from build123d import *

# Parameters (mm, degrees)
F0_R     = 2
F0_R_2   = 39
F0_R_3   = 34
F1_DEPTH = 5
F2_R     = 38
F2_R_2   = 47
F3_DEPTH = 0.5


# Not quite as in the source:
# - a fillet or chamfer that OpenCascade refuses, or shapes differently, is made with other operations: its cross-section is extruded or revolved along the edge and cut away or added


with BuildPart() as f1:
    # F0 (on Front) → F1 (new body)
    with BuildSketch(Plane.XZ):
        with BuildLine():
            ThreePointArc((129, -48), (177, 0), (129, 48))
            Line((129, 48), (0, 48))
            Line((0, 48), (-129, 48))
            ThreePointArc((-129, 48), (-177, 0), (-129, -48))
            Line((-129, -48), (0, -48))
            Line((0, -48), (129, -48))
        make_face()
        with Locations((-129, -42)):
            Circle(F0_R, mode=Mode.SUBTRACT)
        with Locations((-42, -42)):
            Circle(F0_R, mode=Mode.SUBTRACT)
        with Locations((42, -42)):
            Circle(F0_R, mode=Mode.SUBTRACT)
        with Locations((129, -42)):
            Circle(F0_R, mode=Mode.SUBTRACT)
        with Locations((-171, 0)):
            Circle(F0_R, mode=Mode.SUBTRACT)
        with Locations((-129, 0)):
            Circle(F0_R_2, mode=Mode.SUBTRACT)
        with Locations((-87, 0)):
            Circle(F0_R, mode=Mode.SUBTRACT)
        with Locations((-42, 0)):
            Circle(F0_R_3, mode=Mode.SUBTRACT)
        with Locations((-129, 42)):
            Circle(F0_R, mode=Mode.SUBTRACT)
        with Locations((-42, 42)):
            Circle(F0_R, mode=Mode.SUBTRACT)
        Circle(F0_R, mode=Mode.SUBTRACT)
        with Locations((42, 0)):
            Circle(F0_R_3, mode=Mode.SUBTRACT)
        with Locations((87, 0)):
            Circle(F0_R, mode=Mode.SUBTRACT)
        with Locations((129, 0)):
            Circle(F0_R_2, mode=Mode.SUBTRACT)
        with Locations((171, 0)):
            Circle(F0_R, mode=Mode.SUBTRACT)
        with Locations((42, 42)):
            Circle(F0_R, mode=Mode.SUBTRACT)
        with Locations((129, 42)):
            Circle(F0_R, mode=Mode.SUBTRACT)
    extrude(amount=F1_DEPTH)

    # F2 (on face) → F3 (cut)
    with BuildSketch(Plane.XZ.offset(5)):
        with Locations((42, 0)):
            Circle(F2_R)
        with Locations((-42, 0)):
            Circle(F2_R)
        with Locations((129, 0)):
            Circle(F2_R_2)
        with Locations((-129, 0)):
            Circle(F2_R_2)
    extrude(amount=-F3_DEPTH, mode=Mode.SUBTRACT)

    # F4: chamfer of 3 on 4 edges, made by hand

    # F4_s1 → F4_t2 (revolve, cut)
    with BuildSketch(Plane.XY):
        Polygon((-87, 0), (-90, -3), (-90, 0), align=None)
    revolve(axis=Axis((-129, 0, 0), (0, -1, 0)), mode=Mode.SUBTRACT)

    # F4_s3 → F4_t4 (revolve, cut)
    with BuildSketch(Plane.XY):
        Polygon((-5, 0), (-8, -3), (-8, 0), align=None)
    revolve(axis=Axis((-42, 0, 0), (0, -1, 0)), mode=Mode.SUBTRACT)

    # F4_s5 → F4_t6 (revolve, cut)
    with BuildSketch(Plane.XY):
        Polygon((79, 0), (76, -3), (76, 0), align=None)
    revolve(axis=Axis((42, 0, 0), (0, -1, 0)), mode=Mode.SUBTRACT)

    # F4_s7 → F4_t8 (revolve, cut)
    with BuildSketch(Plane.XY):
        Polygon((171, 0), (168, -3), (168, 0), align=None)
    revolve(axis=Axis((129, 0, 0), (0, -1, 0)), mode=Mode.SUBTRACT)


solid = f1.part
The model under review builds one solid part; all positions refer to its coordinate system, in mm. A direction names the side the tool comes from. Give positions to 0.01 mm unless a question says otherwise; leave off trailing zeros. Answer in a Markdown table with one row per item. Add a question column.
1. Add section A-A on z = 25. Count the separate pieces of the cut face and the enclosed holes in it, plus the area to 3 significant figures.
2. Machinability: for faces 5 (the cylindrical face through (-75.967, -3.74, 1.495)), 6 (the cylindrical face through (-175.955, -4.754, 2.067)), which of the approach directions +Z, -Z, +X, -X, +Y, -Y give a long, thin tool a straight path to every point of the face, cutting with its end or side? Answer none if there is none.
3. To check wall thickness, follow line 1 along X through (y, z) = (-2.7, 10); line 2 along Z through (x, y) = (87, -1.55); line 3 along X through (y, z) = (-2.75, 2.5). State the ranges of each line that lie inside material, in increasing order.
4. For pin 1 Ø3.5 at (x, z) = (-42, 42) entering from +Y; pin 2 Ø6.5 at (x, z) = (87, 0) entering from -Y; pin 3 Ø1 at (x, z) = (140.5, 37.5) entering from +Y; pin 4 Ø1.5 at (y, z) = (-1.5, 29.5) entering from +X, all flat-tipped, find the tip position at first contact; note any pin that passes through.
5. Mouldability with a two-part tool opening along X and no side actions: class faces 1 (the cylindrical face through (77.102, -4.754, -14.554)), 2 (the cylindrical face through (176.99, -2.46, -1.06)), 3 (the flat face through (-1, -5, -3)), 4 (the conical face through (74.57, -2.85, 10.26)) as released by +X, released by -X, zero draft, split by the parting line, or undercut.
The answers:
| question | item | result |
|---|---|---|
| 1 | separate pieces | 5 |
| 1 | enclosed holes | 0 |
| 1 | area | 561 mm2 |
| 2 | face 5 | +Y, -Y |
| 2 | face 6 | -Y |
| 3 | line 1 | -175.95 to -167.01, -90.99 to -74.81, -9.19 to 9.19, 74.81 to 90.99, 167.01 to 175.95 |
| 3 | line 2 | -48 to -2, 2 to 48 |
| 3 | line 3 | -176.93 to -168.17, -89.83 to -76.16, -7.84 to 7.84, 76.16 to 89.83, 168.17 to 176.93 |
| 4 | pin 1 | through |
| 4 | pin 2 | y = -4.5 |
| 4 | pin 3 | y = -2.28 |
| 4 | pin 4 | x = 167.44 |
| 5 | face 1 | undercut |
| 5 | face 2 | released by +X |
| 5 | face 3 | zero draft |
| 5 | face 4 | undercut |
